Source: CAD feature listing. Evaluate the final solid. Frame: model axes, mm. A direction names the side the tool comes from. Give positions to 0.01 mm unless a question says otherwise; leave off trailing zeros. Order: outer loops, then holes, each group sorted by start corner. A loop starts at its lowest first (then second) coordinate and runs counter-clockwise, first axis right, second up.
from build123d import *

# Parameters (mm, degrees)
SKETCH1_W                       = 87.884
SKETCH1_H                       = 94.488
BOSS_EXTRUDE1_DEPTH             = 139.446
SKETCH2_R                       = 8.5
BOSS_EXTRUDE2_DEPTH             = 55.118
SKETCH3_R                       = 39.6875
BOSS_EXTRUDE3_DEPTH             = 176.022
SKETCH4_W                       = 87.884
SKETCH4_H                       = 24.892
BOSS_EXTRUDE4_DEPTH             = 21.844
BOSS_EXTRUDE5_DEPTH             = 5.842
NOT_VERIFIED_EXTRUDE_DEPTH      = 10.033
SKETCH8_R                       = 2.75
CUT_EXTRUDE2_DEPTH              = 25.4
SKETCH7_R                       = 12.7
CHANGE_FOR_OPPOSITE_MOTOR_DEPTH = 339.432482365
SKETCH9_R                       = 3
CUT_EXTRUDE3_DEPTH              = 12.7
SKETCH10_R                      = 8.5725
BOSS_EXTRUDE6_DEPTH             = 6.096
SKETCH14_R                      = 1.5
CUT_EXTRUDE4_DEPTH              = 25.4
BOSS_EXTRUDE7_START             = 9.398
SKETCH11_R                      = 8.5
BOSS_EXTRUDE7_DEPTH             = 9.398
SKETCH12_R                      = 21.02690679
BOSS_EXTRUDE8_DEPTH             = 50.4825
SKETCH13_W                      = 14.986
SKETCH13_H                      = 14.986
BOSS_EXTRUDE9_DEPTH             = 6.35
BRAKE_AND_END_CAP_DEPTH         = 27.686
BRAKE_AND_END_CAP_DEPTH_BACK    = 9.398
SKETCH15_R                      = 41.275


with BuildPart() as part:
    # Sketch1 → Boss-Extrude1 (new body)
    with BuildSketch(Plane.XY):
        Rectangle(SKETCH1_W, SKETCH1_H)
    extrude(amount=-BOSS_EXTRUDE1_DEPTH)

    # Sketch2 → Boss-Extrude2 (add)
    with BuildSketch(Plane(origin=(43.942, 0, 0), x_dir=(0, 0, -1), z_dir=(1, 0, 0))):
        with Locations(Location((41.91, 5.6388, 0), (0, 0, 270))):
            Circle(SKETCH2_R)
    extrude(amount=BOSS_EXTRUDE2_DEPTH)

    # Sketch3 → Boss-Extrude3 (add)
    with BuildSketch(Plane(origin=(0, 0, -139.446), x_dir=(-1, 0, 0), z_dir=(0, 0, -1))):
        with Locations(Location((0, 27.686, 0), (0, 0, 150.475215814))):
            Circle(SKETCH3_R)
    extrude(amount=BOSS_EXTRUDE3_DEPTH)

    # Sketch4 → Boss-Extrude4 (add)
    with BuildSketch(Plane.XY.offset(-139.446)):
        with Locations((0, 59.69)):
            Rectangle(SKETCH4_W, SKETCH4_H)
    extrude(amount=BOSS_EXTRUDE4_DEPTH)

    # Sketch5 → Boss-Extrude5 (add, symmetric)
    with BuildSketch(Plane(origin=(0, 0, 0), x_dir=(0, 0, -1), z_dir=(1, 0, 0))):
        Polygon((41.00062989, 47.244), (117.602, 68.118364724), (117.602, 47.244), align=None)
    extrude(amount=BOSS_EXTRUDE5_DEPTH, both=True)

    # Sketch6 → not verified extrude (add)
    with BuildSketch(Plane(origin=(43.942, 0, 0), x_dir=(0, 0, -1), z_dir=(1, 0, 0))):
        with BuildLine():
            Line((67.062792106, 10.685062506), (77.582823134, 7.605402716))
            ThreePointArc((77.582823134, 7.605402716), (103.428106849, -7.84112489), (73.318774576, -7.88601899))
            Line((73.318774576, -7.88601899), (62.51780348, -9.640144719))
            ThreePointArc((62.51780348, -9.640144719), (16.874294712, 11.237119098), (67.062792106, 10.685062506))
        make_face()
    extrude(amount=NOT_VERIFIED_EXTRUDE_DEPTH)

    # Sketch8 → Cut-Extrude2 (cut)
    with BuildSketch(Plane(origin=(0, 0, -139.446), x_dir=(-1, 0, 0), z_dir=(0, 0, -1))):
        with Locations((-35.56, 63.246)):
            Circle(SKETCH8_R)
        with Locations((35.56, 63.246)):
            Circle(SKETCH8_R)
        with Locations((35.56, -7.874)):
            Circle(SKETCH8_R)
        with Locations((-35.56, -7.874)):
            Circle(SKETCH8_R)
    extrude(amount=-CUT_EXTRUDE2_DEPTH, mode=Mode.SUBTRACT)

    # Sketch7 → change for opposite motor (cut, through all)
    with BuildSketch(Plane.XY):
        with Locations((14.097, -47.244)):
            Circle(SKETCH7_R)
    extrude(amount=-CHANGE_FOR_OPPOSITE_MOTOR_DEPTH, mode=Mode.SUBTRACT)

    # Sketch9 → Cut-Extrude3 (cut)
    with BuildSketch(Plane.XZ.offset(47.244)):
        with Locations((-8.001, -7.9756)):
            Circle(SKETCH9_R)
        with Locations((-8.001, -68.3768)):
            Circle(SKETCH9_R)
        with Locations((-8.001, -128.778)):
            Circle(SKETCH9_R)
        with Locations((36.449, -128.778)):
            Circle(SKETCH9_R)
        with Locations((36.449, -68.3768)):
            Circle(SKETCH9_R)
        with Locations((36.449, -7.9756)):
            Circle(SKETCH9_R)
    extrude(amount=-CUT_EXTRUDE3_DEPTH, mode=Mode.SUBTRACT)

    # Sketch10 → Boss-Extrude6 (add)
    with BuildSketch(Plane.XZ.offset(47.244)):
        with Locations(Location((-32.639, -31.496, 0), (0, 0, 180))):
            Circle(SKETCH10_R)
        with Locations(Location((-32.639, -104.4448, 0), (0, 0, 180))):
            Circle(SKETCH10_R)
    extrude(amount=BOSS_EXTRUDE6_DEPTH)

    # Sketch14 → Cut-Extrude4 (cut)
    with BuildSketch(Plane(origin=(0, 0, -315.468), x_dir=(-1, 0, 0), z_dir=(0, 0, -1))):
        with Locations((-26.5, 27.686)):
            Circle(SKETCH14_R)
        with Locations((26.5, 27.686)):
            Circle(SKETCH14_R)
    extrude(amount=-CUT_EXTRUDE4_DEPTH, mode=Mode.SUBTRACT)

    # Sketch11 → Boss-Extrude7 (add)
    with BuildSketch(Plane.ZY.offset(43.942).offset(BOSS_EXTRUDE7_START)):
        with BuildLine():
            Line((-77.582823134, 7.605402716), (-67.062792106, 10.685062506))
            ThreePointArc((-67.062792106, 10.685062506), (-16.874294712, 11.237119098), (-62.51780348, -9.640144719))
            Line((-62.51780348, -9.640144719), (-73.318774576, -7.88601899))
            ThreePointArc((-73.318774576, -7.88601899), (-103.428106849, -7.84112489), (-77.582823134, 7.605402716))
        make_face()
        with Locations(Location((-41.91, 5.6388, 0), (0, 0, 270))):
            Circle(SKETCH11_R, mode=Mode.SUBTRACT)
    extrude(amount=-BOSS_EXTRUDE7_DEPTH)

    # Sketch12 → Boss-Extrude8 (add, symmetric)
    with BuildSketch(Plane(origin=(0, 0, 0), x_dir=(0, 0, -1), z_dir=(1, 0, 0))):
        with Locations(Location((278.212507153, 26.972524542, 0), (0, 0, 180))):
            Circle(SKETCH12_R)
    extrude(amount=BOSS_EXTRUDE8_DEPTH, both=True)

    # Sketch13 → Boss-Extrude9 (add)
    with BuildSketch(Plane(origin=(0, 0, -315.468), x_dir=(-1, 0, 0), z_dir=(0, 0, -1))):
        with Locations((0, 27.686)):
            Rectangle(SKETCH13_W, SKETCH13_H)
    extrude(amount=BOSS_EXTRUDE9_DEPTH)

    # Sketch15 → brake and end cap (add, two sides: drawn at the far end of the back side and taken through both)
    with BuildSketch(Plane(origin=(0, 0, -315.468), x_dir=(-1, 0, 0), z_dir=(0, 0, -1)).offset(-BRAKE_AND_END_CAP_DEPTH_BACK)):
        with Locations((0, 27.686)):
            Circle(SKETCH15_R)
    extrude(amount=BRAKE_AND_END_CAP_DEPTH + BRAKE_AND_END_CAP_DEPTH_BACK)


solid = part.part
1) Pull-direction query (Z, two-part tool) for faces 1 (the face through (1, 28, -343.154)), 2 (the face through (-48.707, 12.187, -17.106)), 3 (the face through (-48.707, -8.775, -67.843)), 4 (the face through (5.842, 53, -97)); classes: +Z half, -Z half, draft (parallel to the pull), parting line (faces both ways), or undercut.
Checks:
face 1: -Z half
face 2: undercut
face 3: undercut
face 4: draft
2) Section query B-B on z = -292. Output: boundary loops of the cut face in (x, y) (1 decimal), and give its area (3 significant figures).
Checks:
outline: (-50.5, 11.1) - (-36.1, 11.1) arc R39.7 ccw to (36.1, 11.1) - (50.5, 11.1) - (50.5, 42.8) - (36.7, 42.8) arc R39.7 ccw to (-36.7, 42.8) - (-50.5, 42.8) - close
area: 5,700 mm2
3) Reachability of faces 5 (the face through (-43.642, 6.125, -280.95)), 6 (the face through (48.888, 9.167, -72.249)), 7 (the face through (-50.482, 27, -279)), 8 (the face through (9, 60, -117.602)), 9 (the face through (-8, -34.544, -68)) from +Z, -Z, +X, -X, +Y, -Y: full face, straight path, thin tool, end or side. Return the list, or none.
Checks:
face 5: -X
face 6: +X, +Y
face 7: -Z, -X, +Y, -Y
face 8: +Z, +Y
face 9: -Y
4) Ray query, L1, parallel to Y at x = -35.56, z = -128.5; L2, parallel to Y at x = 35, z = -131; L3, parallel to Z at x = 43.5, y = 62.5. Return the intervals inside material, ascending.
Checks:
L1: y = -47.24 to -10.62, -5.12 to 60.5, 66 to 72.14
L2: y = -34.54 to -10.57, -5.18 to 60.55, 65.94 to 72.14
L3: z = -139.45 to -117.6
5) Section query A-A on y = -39. Output: boundary loops of the cut face in (x, z).
Checks:
outline: (-43.94, -139.45) - (4.44, -139.45) - (4.44, 0) - (-43.94, 0) - close; (23.76, -139.45) - (43.94, -139.45) - (43.94, 0) - (23.76, 0) - close; hole circle Ø6 at (-8, -128.78); hole circle Ø6 at (-8, -68.38); hole circle Ø6 at (-8, -7.98); hole circle Ø6 at (36.45, -128.78); hole circle Ø6 at (36.45, -68.38); hole circle Ø6 at (36.45, -7.98)
6) First-contact query: pin 1 Ø12.5 at (y, z) = (32.5, -276.5) entering from +X; pin 2 Ø7 at (x, z) = (36.45, -7.98) entering from +Y; pin 3 Ø5 at (x, y) = (-35.56, 63.246) entering from -Z; pin 4 Ø1.8 at (x, z) = (-7.5, -9) entering from -Y. Flat tips, straight axial feed; report the tip coordinate or a pass-through.
Checks:
pin 1: stops at x = 50.48
pin 2: stops at y = 47.24
pin 3: passes through
pin 4: stops at y = -34.54
7) Section query D-D on y = 19.5. Output: boundary loops of the cut face in (x, z) (1 decimal), and give its area (3 significant figures).
Checks:
outline: (-53.3, -63.5) - (-43.9, -63.5) - (-43.9, -139.4) - (-38.8, -139.4) - (-38.8, -258.6) - (-50.5, -258.6) - (-50.5, -297.9) - (-38.8, -297.9) - (-38.8, -306.1) - (-40.5, -306.1) - (-40.5, -343.2) - (40.5, -343.2) - (40.5, -306.1) - (38.8, -306.1) - (38.8, -297.9) - (50.5, -297.9) - (50.5, -258.6) - (38.8, -258.6) - (38.8, -139.4) - (43.9, -139.4) - (43.9, -63.5) - (54, -63.5) - (54, -20.3) - (43.9, -20.3) - (43.9, 0) - (-43.9, 0) - (-43.9, -20.3) - (-53.3, -20.3) - close
area: 30,000 mm2
8) Section query C-C on y = 52.5. Output: boundary loops of the cut face in (x, z), and give its area (3 significant figures).
Checks:
outline: (-43.94, -139.45) - (-30.97, -139.45) - (-30.97, -306.07) - (-32.98, -306.07) - (-32.98, -343.15) - (32.98, -343.15) - (32.98, -306.07) - (30.97, -306.07) - (30.97, -139.45) - (43.94, -139.45) - (43.94, -117.6) - (5.84, -117.6) - (5.84, -60.29) - (-5.84, -60.29) - (-5.84, -117.6) - (-43.94, -117.6) - close
area: 15,400 mm2
